Can you work these out from the model? Positions are in its coordinate system, mm. A direction names the side the tool comes from. Give positions to 0.01 mm unless a question says otherwise; leave off trailing zeros. Loops run counter-clockwise (first coordinate to the right, second up) from the corner with the lowest first, then second, coordinate; pieces in that order, holes last. Notation, with made-up numbers: M -33,5.25 L -8,5.25 A23 cw -8,23.25 Z; hole C -36,-30 d5. An arc over 180 degrees is marked long. One line per item, written item: value. Start each with the question number.
from build123d import *
from OCP.BRepFilletAPI import BRepFilletAPI_MakeChamfer

# Parameters (mm, degrees)
ESQUISSE1_W             = 60
ESQUISSE1_H             = 47
BOSS_EXTRU_1_DEPTH      = 23
ESQUISSE2_W             = 50
ESQUISSE2_H             = 45
ENL_V_MAT_EXTRU_1_DEPTH = 1
ESQUISSE3_W             = 48
ESQUISSE3_H             = 43
ENL_V_MAT_EXTRU_2_DEPTH = 3
ENL_V_MAT_EXTRU_3_DEPTH = 21
ESQUISSE5_R             = 7.5
ENL_V_MAT_EXTRU_4_DEPTH = 51
ESQUISSE8_W             = 2
ESQUISSE8_H             = 15
ENL_V_MAT_EXTRU_5_DEPTH = 17
ESQUISSE9_R             = 2
ENL_V_MAT_EXTRU_6_DEPTH = 80.61155695
CHANFREIN1_SIZE         = 1
CHANFREIN1_SIZE2        = 1.428148007
ESQUISSE10_W            = 5
ESQUISSE10_H            = 10
ENL_V_MAT_EXTRU_7_DEPTH = 1


with BuildPart() as part:
    # Esquisse1 → Boss.-Extru.1 (new body)
    with BuildSketch(Plane.XY):
        with Locations((30, 23.5)):
            Rectangle(ESQUISSE1_W, ESQUISSE1_H)
    extrude(amount=BOSS_EXTRU_1_DEPTH)

    # Esquisse2 → Enlèv. mat.-Extru.1 (cut)
    with BuildSketch(Plane.XY.offset(23)):
        with Locations((26, 23.5)):
            Rectangle(ESQUISSE2_W, ESQUISSE2_H)
    extrude(amount=-ENL_V_MAT_EXTRU_1_DEPTH, mode=Mode.SUBTRACT)

    # Esquisse3 → Enlèv. mat.-Extru.2 (cut)
    with BuildSketch(Plane.XY.offset(22)):
        with Locations((26, 23.5)):
            Rectangle(ESQUISSE3_W, ESQUISSE3_H)
    extrude(amount=-ENL_V_MAT_EXTRU_2_DEPTH, mode=Mode.SUBTRACT)

    # Esquisse4 → Enlèv. mat.-Extru.3 (cut)
    with BuildSketch(Plane.XY.offset(23)):
        Polygon((60, 43.5), (58.5, 45), (57, 43.5), (57, 3.5), (58.5, 2), (60, 3.5), align=None)
    extrude(amount=-ENL_V_MAT_EXTRU_3_DEPTH, mode=Mode.SUBTRACT)

    # Esquisse5 → Enlèv. mat.-Extru.4 (cut)
    with BuildSketch(Plane(origin=(57, 0, 0), x_dir=(0, 0, -1), z_dir=(1, 0, 0))):
        with Locations(Location((-9.5, 31.5, 0), (0, 0, 90))):
            Circle(ESQUISSE5_R)
        with Locations(Location((-9.5, 15.5, 0), (0, 0, 90))):
            Circle(ESQUISSE5_R)
    extrude(amount=-ENL_V_MAT_EXTRU_4_DEPTH, mode=Mode.SUBTRACT)

    # Esquisse8 → Enlèv. mat.-Extru.5 (cut)
    with BuildSketch(Plane.XY.offset(19)):
        with Locations((6, 31.5)):
            Rectangle(ESQUISSE8_W, ESQUISSE8_H)
        with Locations((6, 15.5)):
            Rectangle(ESQUISSE8_W, ESQUISSE8_H)
    extrude(amount=-ENL_V_MAT_EXTRU_5_DEPTH, mode=Mode.SUBTRACT)

    # Esquisse9 → Enlèv. mat.-Extru.6 (cut, through all)
    with BuildSketch(Plane(origin=(0, 0, 0), x_dir=(-1, 0, 0), z_dir=(0, 0, -1))):
        with Locations((-48, 43)):
            Circle(ESQUISSE9_R)
        with Locations((-4, 43)):
            Circle(ESQUISSE9_R)
        with Locations((-4, 4)):
            Circle(ESQUISSE9_R)
        with Locations((-48, 4)):
            Circle(ESQUISSE9_R)
    extrude(amount=-ENL_V_MAT_EXTRU_6_DEPTH, mode=Mode.SUBTRACT)

    # Chanfrein1: one chamfer whose edges measure the first distance from different faces: ONE call of the kernel's chamfer builder (chamfer() names one face for all edges)
    chanfrein1_edges_1 = [part.edges().sort_by_distance(p)[0] for p in [
        (50, 43, 0),
        (6, 43, 0),
        (6, 4, 0),
    ]]
    chanfrein1_side_1 = [part.faces().sort_by_distance(p)[0] for p in [
        (30.072592492, 23.5, 0),
    ]]
    chanfrein1_edges_2 = [part.edges().sort_by_distance(p)[0] for p in [
        (50, 4, 0),
    ]]
    chanfrein1_side_2 = [part.faces().sort_by_distance(p)[0] for p in [
        (50, 4, 9.5),
    ]]
    chanfrein1 = BRepFilletAPI_MakeChamfer(part.part.solid().wrapped)
    for e in chanfrein1_edges_1:
        chanfrein1.Add(CHANFREIN1_SIZE, CHANFREIN1_SIZE2, e.wrapped, chanfrein1_side_1[0].wrapped)  # the first distance lies on this face
    for e in chanfrein1_edges_2:
        chanfrein1.Add(CHANFREIN1_SIZE, CHANFREIN1_SIZE2, e.wrapped, chanfrein1_side_2[0].wrapped)  # the first distance lies on this face
    add(Compound.cast(chanfrein1.Shape()), mode=Mode.REPLACE)

    # Esquisse10 → Enlèv. mat.-Extru.7 (cut)
    with BuildSketch(Plane(origin=(57, 0, 0), x_dir=(0, 0, -1), z_dir=(1, 0, 0))):
        with Locations((-9.5, 22.68303286)):
            Rectangle(ESQUISSE10_W, ESQUISSE10_H)
    extrude(amount=-ENL_V_MAT_EXTRU_7_DEPTH, mode=Mode.SUBTRACT)


solid = part.part
Q1. If we section it at A-A, the plane y = 25.5: Write out the boundary of the cut face in (x, z).
Q2. If we mould it in two halves opening along X, with no side actions, what happens to faces 1 (the face through (56, 23.5, 9.5)), 2 (the face through (30, 47, 11)), 3 (the face through (57.8, 44.3, 12.6))? For each: released by +X, released by -X, zero draft, split by the parting line, or undercut.
Q3. If we section it at B-B, the plane x = 35: Write out the boundary of the cut face in (y, z).
Q4. For P1, Ø1, axis at y = 41.5, z = 18, coming from the +X side; P2, Ø2, axis at x = 49, y = 44.5, coming from the +Z side; P3, Ø5, axis at x = 4, y = 43, coming from the -Z side, each with a flat end and sliding along its axis, tell me the tip position at first contact or that it passes through.
Q5. Which directions (+Z, -Z, +X, -X, +Y, -Y) give clear straight access to the entire face, cutting with the end or side of a thin tool? Please do faces 4 (the face through (4, 41, 10)), 5 (the face through (6, 39, 11)), 6 (the face through (57, 24, 4)).
Q6. I need wall thicknesses on line 1 along X through (y, z) = (4, 15); line 2 along X through (y, z) = (16, 18.5); line 3 along Z through (x, y) = (17.5, 31.5). Which ranges of each line are inside material? Lowest first, please.
Q7. If we section it at C-C, the plane z = 13.5: Give the number of separate pieces and of enclosed holes in the cut face, plus the area to 3 significant figures.
Response:
1. outline: M 0,0 L 60,0 L 60,2 L 57,2 L 57,5 L 7,5 L 7,2 L 5,2 L 5,19 L 2,19 L 2,22 L 1,22 L 1,23 L 0,23 Z; M 7,14 L 57,14 L 57,23 L 51,23 L 51,22 L 50,22 L 50,19 L 7,19 Z
2. face 1: released by +X
2. face 2: zero draft
2. face 3: undercut
3. outline: M 0,0 L 47,0 L 47,23 L 46,23 L 46,22 L 45,22 L 45,19 L 2,19 L 2,22 L 1,22 L 1,23 L 0,23 Z; hole C 15.5,9.5 d15; hole C 31.5,9.5 d15
4. P1: x = 57
4. P2: z = 22
4. P3: z = 0.71
5. face 4: +Z, -Z
5. face 5: +Z
5. face 6: +Z, +X
6. line 1: 0 to 2, 6 to 46, 50 to 57
6. line 2: 0 to 5, 7 to 57
6. line 3: 0 to 2, 17 to 19
7. separate pieces: 1
7. enclosed holes: 4
7. area: 1,320 mm^2
